Part model, mm, in its own coordinate system. A direction names the side the tool comes from. Round coordinates to 2 decimals unless told otherwise and drop trailing zeros. Write each loop counter-clockwise with the first axis right and the second up, starting at its lowest first coordinate (ties: lowest second). Pieces come first, ordered by that corner, then holes.
```python
from build123d import *

# Parameters (mm, degrees)
SKETCH_1_W          = 20
SKETCH_1_H          = 10
SKETCH_1_W_2        = 17
SKETCH_1_H_2        = 7
EXTRUDE_1_DEPTH     = 370
SKETCH_2_R          = 7
CUT_EXTRUDE_1_DEPTH = 10
EXTRUDE_2_DEPTH     = 10


with BuildPart() as part:
    # 草图1 → 凸台-拉伸1 (new body)
    with BuildSketch(Plane.XY):
        Rectangle(SKETCH_1_W, SKETCH_1_H)
        Rectangle(SKETCH_1_W_2, SKETCH_1_H_2, mode=Mode.SUBTRACT)
    extrude(amount=EXTRUDE_1_DEPTH)

    # 草图2 → 切除-拉伸1 (cut)
    with BuildSketch(Plane(origin=(0, 5, 0), x_dir=(1, 0, 0), z_dir=(0, 1, 0))):
        with Locations(Location((0, -15, 0), (0, 0, 270))):
            Circle(SKETCH_2_R)
        with Locations(Location((0, -335, 0), (0, 0, 270))):
            Circle(SKETCH_2_R)
    extrude(amount=-CUT_EXTRUDE_1_DEPTH, mode=Mode.SUBTRACT)

    # 草图3 → 凸台-拉伸2 (add)
    with BuildSketch(Plane(origin=(0, 5, 0), x_dir=(1, 0, 0), z_dir=(0, 1, 0))):
        with BuildLine():
            Line((-10, -370), (10, -370))
            ThreePointArc((10, -370), (0, -380), (-10, -370))
        make_face()
    extrude(amount=-EXTRUDE_2_DEPTH)


solid = part.part
```
Q1. Cut at A-A on x = 0. Write the cut outline in (y, z), plus the area to 3 significant figures.
Values follow:
outline: (-5, 0) - (-3.5, 0) - (-3.5, 8) - (-5, 8) - close; (-5, 22) - (-3.5, 22) - (-3.5, 328) - (-5, 328) - close; (-5, 342) - (-3.5, 342) - (-3.5, 370) - (3.5, 370) - (3.5, 342) - (5, 342) - (5, 380) - (-5, 380) - close; (3.5, 0) - (5, 0) - (5, 8) - (3.5, 8) - close; (3.5, 22) - (5, 22) - (5, 328) - (3.5, 328) - close
area: 1,130 mm2
Q2. Cut at B-B on z = 15. Write the cut outline in (x, y).
Values follow:
outline: (-10, -5) - (-7, -5) - (-7, -3.5) - (-8.5, -3.5) - (-8.5, 3.5) - (-7, 3.5) - (-7, 5) - (-10, 5) - close; (7, -5) - (10, -5) - (10, 5) - (7, 5) - (7, 3.5) - (8.5, 3.5) - (8.5, -3.5) - (7, -3.5) - close
Q3. Drop flat-ended pins along their axis: pin 1 (5.5 mm diameter, centred on x = -0.5, y = 0, fed in from -Z); pin 2 (4 mm diameter, centred on x = -4.5, y = -3.5, fed in from +Z). Give the stop position or say it passes through.
Values follow:
pin 1: stops at z = 370
pin 2: stops at z = 379.68
Q4. Which spindle directions (+Z, -Z, +X, -X, +Y, -Y) get a long thin tool onto all of the face, cutting with end or side? Do faces 4 (the flat face through (0, 5, 187)), 5 (the flat face through (8.5, 0, 182)). Say none if no direction does.
Values follow:
face 4: +Z, -Z, +X, -X, +Y
face 5: -Z
Q5. Cut at C-C on z = 91.5. Write the cut outline in (x, y).
Values follow:
outline: (-10, -5) - (10, -5) - (10, 5) - (-10, 5) - close; hole (-8.5, -3.5) - (8.5, -3.5) - (8.5, 3.5) - (-8.5, 3.5) - close
Q6. Cut at D-D on y = 1.5. Write the cut outline in (x, z).
Values follow:
outline: (-10, 0) - (-8.5, 0) - (-8.5, 370) - (8.5, 370) - (8.5, 0) - (10, 0) - (10, 370) arc R10 ccw to (-10, 370) - close
Q7. Mould opens along Z. For faces 1 (the flat face through (0, -5, 187)), 2 (the cylindrical face through (0, 4, 8)), 3 (the flat face through (0, 0, 370)) say: +Z half, -Z half, draft (parallel to the pull), parting line (faces both ways), or undercut.
Values follow:
face 1: draft
face 2: undercut
face 3: -Z half
Q8. Wall check: L1, parallel to X at y = -1.25, z = 35; L2, parallel to X at y = 4.65, z = 335; L3, parallel to Y at x = -3.75, z = 141. Give the ranges that are in metal, low to high.
Values follow:
L1: x = -10 to -8.5, 8.5 to 10
L2: x = -10 to -7, 7 to 10
L3: y = -5 to -3.5, 3.5 to 5
